```python
from build123d import *

# Parameters (mm, degrees)
BOSS_EXTRUDE1_DEPTH = 10.16
CUT_LOFT1_START     = 319.572758977
CUT_LOFT1_OUTLINE_W = 1472
CUT_LOFT1_OUTLINE_H = 11.5
CUT_LOFT1_DEPTH     = 38.082840263


# Read off the part's stored shape, not the designer's step: Cut-Loft1
with BuildPart() as part:
    # Sketch1 → Boss-Extrude1 (new body)
    # profile 1 of 2: a face of its own
    with BuildSketch(Plane.XY):
        Polygon((205.715298803, 2062.48), (123.444, 2062.48), (123.444, 2042.16), (41.135649402, 2042.16), (41.135649402, 2062.48), (-41.135649402, 2062.48), (-41.135649402, 2042.16), (-123.444, 2042.16), (-123.444, 2062.48), (-205.715298803, 2062.48), (-205.715298803, 2042.16), (-215.881789204, 2042.16), (-215.881789204, 1953.26), (-205.715298803, 1953.26), (-205.715298803, 1864.36), (-215.881789204, 1864.36), (-215.881789204, 1775.46), (-205.715298803, 1775.46), (-205.715298803, 1686.56), (-215.875298803, 1686.56), (-215.875298803, 1597.66), (-205.715298803, 1597.66), (-205.715298803, 1518.92), (205.715298803, 1518.92), (205.715298803, 1597.66), (215.875298803, 1597.66), (215.875298803, 1686.56), (205.715298803, 1686.56), (205.715298803, 1775.46), (215.881789204, 1775.46), (215.881789204, 1864.36), (205.715298803, 1864.36), (205.715298803, 1953.26), (215.881789204, 1953.26), (215.881789204, 2042.16), (205.715298803, 2042.16), align=None)
    # profile 2 of 2: a face of its own
    with BuildSketch(Plane.XY):
        Polygon((215.881789204, 1518.92), (205.715298803, 1518.92), (-205.715298803, 1518.92), (-215.881789204, 1518.92), (-215.881789204, 1476.636861244), (-402.453189401, 1476.636861244), (-358.672996954, 10.16), (-303.52, 10.16), (-303.52, 0), (-252, 0), (-252, 10.16), (-55.8292, 10.16), (-55.8292, 0), (55.8292, 0), (55.8292, 10.16), (252, 10.16), (252, 0), (303.52, 0), (303.52, 10.16), (358.672996954, 10.16), (402.453189401, 1476.636861244), (215.881789204, 1476.636861244), align=None)
        Polygon((-308.266124544, 132.94397688), (-301.755453134, 226.680843836), (-291.63777305, 225.978101227), (-298.14844446, 132.241234271), align=None, mode=Mode.SUBTRACT)
        Polygon((-289.435698895, 404.053512688), (-279.318018811, 403.350770078), (-285.830533081, 309.587370692), (-295.948213166, 310.290113301), align=None, mode=Mode.SUBTRACT)
        Polygon((-283.630301787, 487.636249721), (-277.115944656, 581.426181539), (-266.998264572, 580.72343893), (-273.512621703, 486.933507112), align=None, mode=Mode.SUBTRACT)
        Polygon((-264.796190418, 758.798850391), (-254.678510334, 758.096107781), (-261.194710324, 664.279643533), (-271.312390408, 664.982386142), align=None, mode=Mode.SUBTRACT)
        Polygon((-252.476436179, 936.171519242), (-242.358756095, 935.468776633), (-248.876798945, 841.625779953), (-258.99447903, 842.328522563), align=None, mode=Mode.SUBTRACT)
        Polygon((301.755453134, 226.680843836), (308.266124544, 132.94397688), (298.14844446, 132.241234271), (291.63777305, 225.978101227), align=None, mode=Mode.SUBTRACT)
        Polygon((279.318018811, 403.350770078), (289.435698895, 404.053512688), (295.948213166, 310.290113301), (285.830533081, 309.587370692), align=None, mode=Mode.SUBTRACT)
        Polygon((277.115944656, 581.426181539), (283.630301787, 487.636249721), (273.512621703, 486.933507112), (266.998264572, 580.72343893), align=None, mode=Mode.SUBTRACT)
        Polygon((254.678510334, 758.096107781), (264.796190418, 758.798850391), (271.312390408, 664.982386142), (261.194710324, 664.279643533), align=None, mode=Mode.SUBTRACT)
        Polygon((242.358756095, 935.468776633), (252.476436179, 936.171519242), (258.99447903, 842.328522563), (248.876798945, 841.625779953), align=None, mode=Mode.SUBTRACT)
        Polygon((-240.15668194, 1113.544188093), (-230.039001856, 1112.841445484), (-236.558887567, 1018.971916374), (-246.676567651, 1019.674658983), align=None, mode=Mode.SUBTRACT)
        Polygon((-227.836927701, 1290.916856945), (-217.719247617, 1290.214114336), (-224.240976188, 1196.318052795), (-234.358656272, 1197.020795404), align=None, mode=Mode.SUBTRACT)
        Polygon((-206.420980822, 1452.880000035), (-211.92306481, 1373.664189215), (-222.040744894, 1374.366931824), (-215.881789204, 1463.040000035), (-205.715298803, 1463.040000035), align=None, mode=Mode.SUBTRACT)
        Polygon((230.039001856, 1112.841445484), (240.15668194, 1113.544188093), (246.676567651, 1019.674658983), (236.558887567, 1018.971916374), align=None, mode=Mode.SUBTRACT)
        Polygon((217.719247617, 1290.214114336), (227.836927701, 1290.916856945), (234.358656272, 1197.020795404), (224.240976188, 1196.318052795), align=None, mode=Mode.SUBTRACT)
        Polygon((205.715298803, 1463.040000035), (215.881789204, 1463.040000035), (222.040744894, 1374.366931824), (211.92306481, 1373.664189215), (206.420980822, 1452.880000035), align=None, mode=Mode.SUBTRACT)
    extrude(amount=BOSS_EXTRUDE1_DEPTH)

    # Cut-Loft1 outline → Cut-Loft1 (cut)
    with BuildSketch(Plane(origin=(0, 0, 0), x_dir=(0.030009511302642098, 0.9995496131915498, 0), z_dir=(0.9995496131915498, -0.030009511302642095, 0)).offset(CUT_LOFT1_START)):
        with Locations((754, 3.75)):
            Rectangle(CUT_LOFT1_OUTLINE_W, CUT_LOFT1_OUTLINE_H)
    cut_loft1 = extrude(amount=CUT_LOFT1_DEPTH, mode=Mode.SUBTRACT)

    # Mirror1: Cut-Loft1 across plane
    add(cut_loft1.mirror(Plane(origin=(0, 0, 0), x_dir=(0, 0, 1), z_dir=(1, 0, 0))), mode=Mode.SUBTRACT)


solid = part.part
```
The model under review builds one solid part; all positions refer to its coordinate system, in mm. A direction names the side the tool comes from. Coordinates: 2 decimals unless noted, no trailing zeros. Write each loop counter-clockwise with the first axis right and the second up, starting at its lowest first coordinate (ties: lowest second). Pieces come first, ordered by that corner, then holes. Notation, with made-up numbers: (36.25, 18.5) - (75.25, 18.5) arc R14 ccw to (75.25, 45.5) - close; hole circle Ø11 at (27, 88.25). An arc over 180 degrees is marked (long way). Answer in a Markdown table with one row per item. Add a question column.
Q1. Consider section D-D on y = 1935.5. Give the boundary of the cut face in (x, z).
Q2. Clearance check with flat-ended pins moving along their axes: pin 1 (3 mm diameter, centred on x = -212, z = 7, fed in from -Y); pin 2 (3 mm diameter, centred on y = 1725.5, z = 7.5, fed in from +X); pin 3 (5 mm diameter, centred on x = 211.5, z = 4.5, fed in from +Y). State where each tip first meets the part, or that it passes through.
Q3. Draft analysis for pull direction Z (two halves, no side actions). For faces 1 (the face through (-6, 1046, 10.16)), 2 (the face through (361, 733, 9.5)), state which applies: +Z half, -Z half, draft (parallel to the pull), parting line (faces both ways), or undercut.
Q4. For faces 3 (the face through (-361, 733, 9.5)), 4 (the face through (-5, 1046, 0)), list the 3-axis set-ups (+Z, -Z, +X, -X, +Y, -Y) from which the entire face can be reached by the end or side of a thin tool; tool diameter is ignored.
Q5. Consider section A-A on y = 880.5. Give the boundary of the cut face in (x, z).
Q6. Consider section C-C on y = 1314. Give the boundary of the cut face in (x, z).
Q7. To check wall thickness, follow line 1 along X through (y, z) = (1363.5, 3.25); line 2 along X through (y, z) = (1403, 2.75); line 3 along X through (y, z) = (1164.5, 7.25). State the ranges of each line that lie inside material, in increasing order. Write a range as from..to.
Q8. Consider section B-B on z = 7.5. Give the number of separate pieces and of enclosed holes in the cut face, then the cut area to 3 significant figures.
Answers below:
| question | item | result |
|---|---|---|
| 1 | outline | (-205.72, 0) - (205.72, 0) - (205.72, 10.16) - (-205.72, 10.16) - close |
| 2 | pin 1 | y = 10.16 |
| 2 | pin 2 | x = 205.72 |
| 2 | pin 3 | y = 2042.16 |
| 3 | face 1 | +Z half |
| 3 | face 2 | -Z half |
| 4 | face 3 | -Z |
| 4 | face 4 | -Z, +X, -X, +Y, -Y |
| 5 | outline | (-384.66, 0) - (-384.25, 0) - (-384.25, 9.5) - (-346.15, 9.5) - (-346.15, 0) - (-256.34, 0) - (-256.34, 10.16) - (-384.66, 10.16) - close; (-246.18, 0) - (246.18, 0) - (246.18, 10.16) - (-246.18, 10.16) - close; (256.34, 0) - (346.15, 0) - (346.15, 9.5) - (384.25, 9.5) - (384.25, 0) - (384.66, 0) - (384.66, 10.16) - (256.34, 10.16) - close |
| 6 | outline | (-397.6, 0) - (-397.27, 0) - (-397.27, 9.5) - (-359.17, 9.5) - (-359.17, 0) - (359.17, 0) - (359.17, 9.5) - (397.27, 9.5) - (397.27, 0) - (397.6, 0) - (397.6, 10.16) - (-397.6, 10.16) - close |
| 7 | line 1 | -399.08..-398.75, -360.65..360.65, 398.75..399.08 |
| 7 | line 2 | -400.25..-399.94, -361.84..-220.05, -209.89..209.89, 220.05..361.84, 399.94..400.25 |
| 7 | line 3 | -393.13..-392.78, -354.68..354.68, 392.78..393.13 |
| 8 | separate pieces | 3 |
| 8 | enclosed holes | 16 |
| 8 | area | 1,240,000 mm² |
